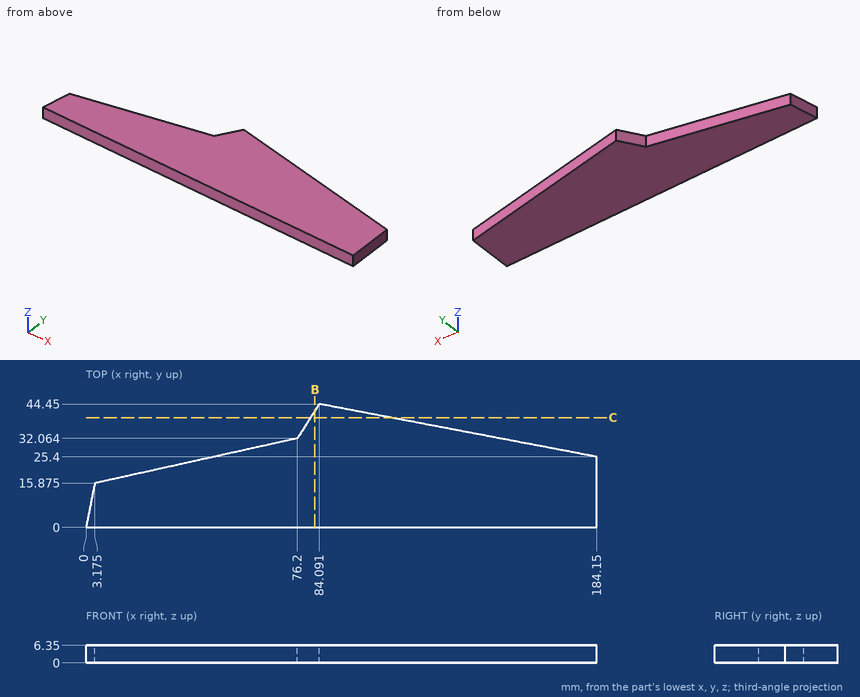
Geometry check sheet. Reference: drawing and pictorial views, mm from the part's lowest x, y, z. Round coordinates to 2 decimals unless told otherwise and drop trailing zeros. Order: outer loops, then holes, each group sorted by start corner. A loop starts at its lowest first (then second) coordinate and runs counter-clockwise, first axis right, second up. Notation, with made-up numbers: (45.25, 53) - (58.25, 53) arc R22 ccw to (58.25, 72) - close; hole circle Ø1 at (-12, -17). An arc over 180 degrees is marked (long way). One line per question, with ' | ' between items. Start each with the question number.
(1) Thickness scan on L1, parallel to Y at x = 157.5, z = 1.5; L2, parallel to Y at x = 109, z = 5.25; L3, parallel to X at y = 2, z = 0.5. Record the ranges inside material, lowest first. Write a range as [from, to].
(2) Sectioned sample at C-C on y = 39.5. Record the cut outline in (x, z).
(3) Sectioned sample at B-B on x = 82.5. Record the cut outline in (y, z).
(4) Depth check by flat-ended pin: pin 1 Ø1.5 at (x, z) = (71, 3) entering from +Y; pin 2 Ø3 at (x, z) = (55, 3.5) entering from +Y. Enter the tip coordinate at first touch or a pass-through.
Conclusion:
1) L1: y = [0, 30.47] | L2: y = [0, 39.71] | L3: x = [0.4, 184.15]
2) outline: (80.94, 0) - (110.09, 0) - (110.09, 6.35) - (80.94, 6.35) - close
3) outline: (0, 0) - (41.95, 0) - (41.95, 6.35) - (0, 6.35) - close
4) pin 1: stops at y = 31.08 | pin 2: stops at y = 27.7
